```python
from build123d import *

# Parameters (mm, degrees)
BOSS_EXTRUDE3_DEPTH = 6.35
SKETCH3_W           = 6.24
SKETCH3_H           = 6.35
BOSS_EXTRUDE4_DEPTH = 6.24
FILLET1_R           = 3.12
SKETCH4_R           = 1
CUT_EXTRUDE1_DEPTH  = 55.454774814
SKETCH5_R           = 1.4224
SKETCH5_R_2         = 1.4732
CUT_EXTRUDE2_DEPTH  = 55.454774814
SKETCH6_W           = 6.24
SKETCH6_H           = 6.35
BOSS_EXTRUDE5_DEPTH = 6.24
SKETCH7_R           = 1
CUT_EXTRUDE3_DEPTH  = 55.454774814
FILLET3_R           = 3.12


with BuildPart() as part:
    # Sketch2 → Boss-Extrude3 (new body)
    with BuildSketch(Plane(origin=(0, 0, 0), x_dir=(1, 0, 0), z_dir=(0, 1, 0))):
        with BuildLine():
            Line((-45, 25.825), (-45, -25.825))
            ThreePointArc((-45, -25.825), (-43.777170811, -28.777170811), (-40.825, -30))
            Line((-40.825, -30), (40.825, -30))
            ThreePointArc((40.825, -30), (43.777170811, -28.777170811), (45, -25.825))
            Line((45, -25.825), (45, 25.825))
            ThreePointArc((45, 25.825), (43.777170811, 28.777170811), (40.825, 30))
            Line((40.825, 30), (-40.825, 30))
            ThreePointArc((-40.825, 30), (-43.777170811, 28.777170811), (-45, 25.825))
        make_face()
        with BuildLine():
            Line((-41.825, -25.825), (-41.825, 25.825))
            ThreePointArc((-41.825, 25.825), (-41.532106781, 26.532106781), (-40.825, 26.825))
            Line((-40.825, 26.825), (40.825, 26.825))
            ThreePointArc((40.825, 26.825), (41.532106781, 26.532106781), (41.825, 25.825))
            Line((41.825, 25.825), (41.825, -25.825))
            ThreePointArc((41.825, -25.825), (41.532106781, -26.532106781), (40.825, -26.825))
            Line((40.825, -26.825), (-40.825, -26.825))
            ThreePointArc((-40.825, -26.825), (-41.532106781, -26.532106781), (-41.825, -25.825))
        make_face(mode=Mode.SUBTRACT)
    extrude(amount=BOSS_EXTRUDE3_DEPTH)

    # Sketch3 → Boss-Extrude4 (add)
    with BuildSketch(Plane(origin=(-7.875425543, 0, 26.825), x_dir=(-1, 0, 0), z_dir=(0, 0, -1))):
        with Locations((-31.660425543, 3.175)):
            Rectangle(SKETCH3_W, SKETCH3_H)
    extrude(amount=BOSS_EXTRUDE4_DEPTH)

    # Fillet1
    fillet1_edges = [part.edges().sort_by_distance(p)[0] for p in [
        (20.665, 3.175, 20.585),
        (26.905, 3.175, 20.585),
    ]]
    fillet(fillet1_edges, radius=FILLET1_R - 0.0001)  # a hair under: the kernel refuses the full size

    # Sketch4 → Cut-Extrude1 (cut, through all)
    with BuildSketch(Plane.XZ):
        with Locations(Location((23.785, 23.705, 0), (0, 0, 270))):
            Circle(SKETCH4_R)
    extrude(amount=-CUT_EXTRUDE1_DEPTH, mode=Mode.SUBTRACT)

    # Sketch5 → Cut-Extrude2 (cut, through all)
    with BuildSketch(Plane.XZ):
        with Locations((-40.824987904, 25.779417466)):
            Circle(SKETCH5_R)
        with Locations((40.825, 25.825)):
            Circle(SKETCH5_R_2)
        with Locations((40.86022953, -25.814867613)):
            Circle(SKETCH5_R_2)
        with Locations((-40.789751469, -25.870570514)):
            Circle(SKETCH5_R_2)
    extrude(amount=-CUT_EXTRUDE2_DEPTH, mode=Mode.SUBTRACT)

    # Sketch6 → Boss-Extrude5 (add)
    with BuildSketch(Plane.XY.offset(-26.825)):
        with Locations((-8.92393673, 3.175)):
            Rectangle(SKETCH6_W, SKETCH6_H)
    extrude(amount=BOSS_EXTRUDE5_DEPTH)

    # Sketch7 → Cut-Extrude3 (cut, through all)
    with BuildSketch(Plane(origin=(0, 0, 0), x_dir=(-1, 0, 0), z_dir=(0, -1, 0))):
        with Locations(Location((8.92393673, 23.705, 0), (0, 0, 90))):
            Circle(SKETCH7_R)
    extrude(amount=-CUT_EXTRUDE3_DEPTH, mode=Mode.SUBTRACT)

    # Fillet3
    fillet3_edges = [part.edges().sort_by_distance(p)[0] for p in [
        (-5.80393673, 3.175, -20.585),
        (-12.04393673, 3.175, -20.585),
    ]]
    fillet(fillet3_edges, radius=FILLET3_R - 0.0001)  # a hair under: the kernel refuses the full size


solid = part.part
```
Could you check a few things on this model? Use its own coordinates, in mm. A direction names the side the tool comes from. Give positions to 0.01 mm unless a question says otherwise; leave off trailing zeros. Loops run counter-clockwise (first coordinate to the right, second up) from the corner with the lowest first, then second, coordinate; pieces in that order, holes last. Notation, with made-up numbers: (-2, -26.5) - (17, -26.5) arc R12 ccw to (17, -11.5) - close; hole circle Ø7 at (47, 11). An arc over 180 degrees is marked (long way). Answer in a Markdown table with one row per item. Add a question column.
Q1. If we section it at C-C (y = 4.75): State how many separate pieces and enclosed holes the cut face has, plus the area to 3 significant figures.
Q2. If we section it at D-D (z = -21.5): List the corners of the cut face in (x, y) for me (3 decimals), plus the area to 3 significant figures.
Q3. Which directions (+Z, -Z, +X, -X, +Y, -Y) give clear straight access to the entire face, cutting with the end or side of a thin tool? Please do faces 1 (the face through (1, 3, -30)), 2 (the face through (26.015, 3.219, 21.523)).
Q4. Please list where these lines run through material, in increasing order: L1, parallel to Z at x = 38, y = 1 (3 decimals); L2, parallel to X at y = 3.25, z = -10 (3 decimals); L3, parallel to X at y = 2.5, z = -22.5 (3 decimals). Write a range as from..to.
Q5. We'd pull the mould along Z, two halves only. Please class faces 3 (the face through (43.809, 3.131, -28.745)), 4 (the face through (45, 3, 0)), 5 (the face through (43.745, 3.131, 28.809)), 6 (the face through (-11.106, 3.219, -21.475)): +Z half, -Z half, draft (parallel to the pull), parting line (faces both ways), or undercut.
Q6. If we section it at B-B (x = -31): List the corners of the cut face in (y, z) for me (3 decimals).
Q7. For pin 1 (6 mm diameter, centred on x = 23, z = 19.5, fed in from +Y), with a flat end and sliding along its axis, tell me the tip position at first contact or that it passes through.
Q8. If we section it at A-A (z = 0.5): List the corners of the cut face in (x, y) for me (3 decimals).
The answers:
| question | item | result |
|---|---|---|
| 1 | separate pieces | 1 |
| 1 | enclosed holes | 3 |
| 1 | area | 955 mm^2 |
| 2 | outline | (-45, 0) - (-41.825, 0) - (-41.825, 6.35) - (-45, 6.35) - close; (-11.131, 0) - (-6.717, 0) - (-6.717, 6.35) - (-11.131, 6.35) - close; (41.825, 0) - (45, 0) - (45, 6.35) - (41.825, 6.35) - close |
| 2 | area | 68.4 mm^2 |
| 3 | face 1 | -Z, +X, -X, +Y, -Y |
| 3 | face 2 | +Y, -Y |
| 4 | L1 | z = -30..-26.825, 26.825..30 |
| 4 | L2 | x = -45..-41.825, 41.825..45 |
| 4 | L3 | x = -45..-41.825, -11.802..-6.046, 41.825..45 |
| 5 | face 3 | -Z half |
| 5 | face 4 | draft |
| 5 | face 5 | +Z half |
| 5 | face 6 | undercut |
| 6 | outline | (0, -30) - (6.35, -30) - (6.35, -26.825) - (0, -26.825) - close; (0, 26.825) - (6.35, 26.825) - (6.35, 30) - (0, 30) - close |
| 7 | pin 1 | stops at y = 6.35 |
| 8 | outline | (-45, 0) - (-41.825, 0) - (-41.825, 6.35) - (-45, 6.35) - close; (41.825, 0) - (45, 0) - (45, 6.35) - (41.825, 6.35) - close |
